Model file for the job. Use its own axes, mm. Round coordinates to 2 decimals unless told otherwise and drop trailing zeros. Loops run counter-clockwise (first coordinate to the right, second up) from the corner with the lowest first, then second, coordinate; pieces in that order, holes last. Notation, with made-up numbers: (-6.5, 16.25) -> (17.5, 16.25) arc R22 ccw to (17.5, 34.25) -> close; hole circle Ø10 at (10.25, 56). An arc over 180 degrees is marked (long way). Use a Markdown table: item, result.
from build123d import *

# Parameters (mm, degrees)
F0_R     = 3.054934
F1_DEPTH = 2


with BuildPart() as f1:
    # F0 (on Top) → F1 (new body)
    with BuildSketch(Plane.XY):
        with BuildLine():
            ThreePointArc((19.515011, 24.16541), (8.491912, 18.245194), (0, 9.055791))
            ThreePointArc((0, 9.055791), (-42.193006, 25.039156), (-79.726435, 0))
            ThreePointArc((-79.726435, 0), (-42.193006, -25.039156), (0, -9.055791))
            ThreePointArc((0, -9.055791), (8.491912, -18.245194), (19.515011, -24.16541))
            ThreePointArc((19.515011, -24.16541), (12.673698, 0), (19.515011, 24.16541))
        make_face()
        with Locations((-60.549479, 6.214748)):
            Circle(F0_R, mode=Mode.SUBTRACT)
    extrude(amount=F1_DEPTH)


solid = f1.part
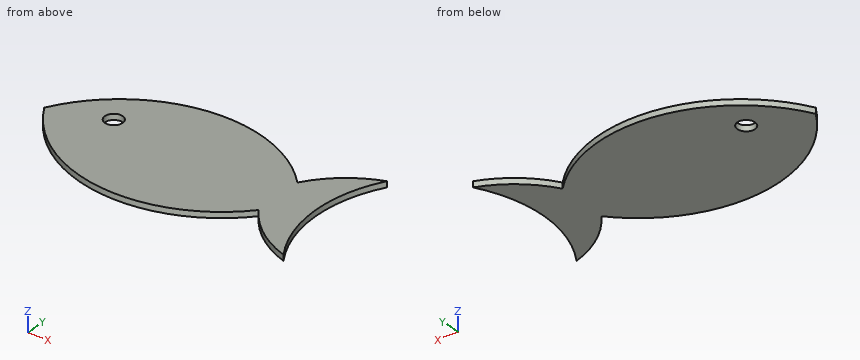
Q1. Band-saw the part on C-C, the plane z = 1.7. Give the cut face in (x, y).
Results list:
| item | result |
|---|---|
| outline | (-79.73, 0) arc R49.31 ccw to (0, -9.06) arc R37.87 ccw to (19.52, -24.17) arc R46.1 cw to (19.52, 24.17) arc R37.87 ccw to (0, 9.06) arc R49.31 ccw to start; hole circle Ø6.11 at (-60.55, 6.21) |
Q2. Band-saw the part on A-A, the plane y = -14. Give the cut face in (x, z), plus the area to 3 significant figures.
Results list:
| item | result |
|---|---|
| outline | (-68.1, 0) -> (-5.15, 0) -> (-5.15, 2) -> (-68.1, 2) -> close; (3.86, 0) -> (14.85, 0) -> (14.85, 2) -> (3.86, 2) -> close |
| area | 148 mm² |
Q3. Band-saw the part on B-B, the plane x = -61.5. Give the cut face in (y, z).
Results list:
| item | result |
|---|---|
| outline | (-18.62, 0) -> (3.31, 0) -> (3.31, 2) -> (-18.62, 2) -> close; (9.12, 0) -> (18.62, 0) -> (18.62, 2) -> (9.12, 2) -> close |
Q4. Band-saw the part on D-D, the plane x = -9. Give the cut face in (y, z), plus the area to 3 significant figures.
Results list:
| item | result |
|---|---|
| outline | (-16.89, 0) -> (16.89, 0) -> (16.89, 2) -> (-16.89, 2) -> close |
| area | 67.5 mm² |
Q5. Flat gauge pin, fed straight in: pin 1 (5 mm diameter, centred on x = -60.55, y = 6.21, fed in from +Z). Where does the tip first touch, or does it go through?
Results list:
| item | result |
|---|---|
| pin 1 | passes through |
Q6. Drill centre lines: L1, parallel to X at y = 13, z = 1.35; L2, parallel to X at y = -14, z = 1.25; L3, parallel to Y at x = -58.5, z = 1. Where is each one in solid material? Low to high. Write a range as from..to.
Results list:
| item | result |
|---|---|
| L1 | x = -69.27..-3.98, 2.97..14.54 |
| L2 | x = -68.1..-5.15, 3.86..14.85 |
| L3 | y = -20.24..3.95, 8.48..20.24 |
